Input: part model. Units: mm. Frame: model coordinates. A direction names the side the tool comes from. Coordinates: 2 decimals unless noted, no trailing zeros. Order: outer loops, then holes, each group sorted by start corner. A loop starts at its lowest first (then second) coordinate and runs counter-clockwise, first axis right, second up. Notation, with made-up numbers: M 14,50 L 62,50 A23 cw 62,84 Z; hole C 29.5,58 d6. An arc over 180 degrees is marked long. Answer in a Markdown table with one row per item.
from build123d import *

# Parameters (mm, degrees)
MAIN_BODY_DEPTH              = 34
SKETCH3_R                    = 3.571875
F_9_32_RIGHT_RAIL_DEPTH      = 1
F_9_32_RIGHT_RAIL_DEPTH_BACK = 39.1
SKETCH4_R                    = 3.571875
F_9_32_LEFT_RAIL_DEPTH       = 34
INNER_HOLLOW_DEPTH           = 21.3
SKETCH6_R                    = 3.571875
F_9_32_TOP_HOLE_DEPTH        = 1
F_9_32_TOP_HOLE_DEPTH_BACK   = 35


with BuildPart() as part:
    # Sketch1 → Main Body (new body)
    with BuildSketch(Plane(origin=(0, 0, 0), x_dir=(1, 0, 0), z_dir=(0, 1, 0))):
        Polygon((0, 0), (38.1, 0), (38.1, 9.525), (9.525, 38.1), (0, 38.1), align=None)
    extrude(amount=MAIN_BODY_DEPTH)

    # Sketch3 → 9/32 Right Rail (cut, two sides)
    with BuildSketch(Plane.XY) as f_9_32_right_rail_sk:
        with Locations((19.05, 17)):
            Circle(SKETCH3_R)
    extrude(amount=F_9_32_RIGHT_RAIL_DEPTH, mode=Mode.SUBTRACT)
    extrude(f_9_32_right_rail_sk.sketch, amount=-F_9_32_RIGHT_RAIL_DEPTH_BACK, mode=Mode.SUBTRACT)

    # Sketch4 → 9/32 Left Rail (cut)
    with BuildSketch(Plane.ZY):
        with Locations((-19.05, 17)):
            Circle(SKETCH4_R)
    extrude(amount=-F_9_32_LEFT_RAIL_DEPTH, mode=Mode.SUBTRACT)

    # Sketch5 → Inner Hollow (cut)
    with BuildSketch(Plane(origin=(0, 27.65, 0), x_dir=(1, 0, 0), z_dir=(0, 1, 0))):
        Polygon((3.175, 28.382403955), (11.208798023, 36.416201977), (36.416201977, 11.208798023), (28.382403955, 3.175), (3.175, 3.175), align=None)
    extrude(amount=-INNER_HOLLOW_DEPTH, mode=Mode.SUBTRACT)

    # Sketch6 → 9/32 Top Hole (cut, two sides)
    with BuildSketch(Plane(origin=(0, 34, 0), x_dir=(1, 0, 0), z_dir=(0, 1, 0))) as f_9_32_top_hole_sk:
        with Locations((11.90625, 11.90625)):
            Circle(SKETCH6_R)
    extrude(amount=F_9_32_TOP_HOLE_DEPTH, mode=Mode.SUBTRACT)
    extrude(f_9_32_top_hole_sk.sketch, amount=-F_9_32_TOP_HOLE_DEPTH_BACK, mode=Mode.SUBTRACT)


solid = part.part
1) Cut plane D-D, the plane z = -19.05. Output: boundary loops of the cut face in (x, y) (3 decimals), and give its area (3 significant figures).
Resolved:
| item | result |
|---|---|
| outline | M 0,0 L 28.575,0 L 28.575,6.35 L 3.175,6.35 L 3.175,13.428 L 0,13.428 Z; M 0,20.572 L 3.175,20.572 L 3.175,27.65 L 28.575,27.65 L 28.575,34 L 0,34 Z |
| area | 408 mm2 |
2) Cut plane B-B, the plane x = 17. Output: boundary loops of the cut face in (y, z) (3 decimals), and give its area (3 significant figures).
Resolved:
| item | result |
|---|---|
| outline | M 0,-30.625 L 6.35,-30.625 L 6.35,-3.175 L 14.075,-3.175 L 14.075,0 L 0,0 Z; M 19.925,-3.175 L 27.65,-3.175 L 27.65,-30.625 L 34,-30.625 L 34,0 L 19.925,0 Z |
| area | 438 mm2 |
3) Material intervals for probe 1 along Y at (x, z) = (13, -19); probe 2 along Y at (x, z) = (2, -19); probe 3 along X at (y, z) = (14.5, -12.5) (3 decimals), sorted ascending.
Resolved:
| item | result |
|---|---|
| probe 1 | y = 0 to 6.35, 27.65 to 34 |
| probe 2 | y = 0 to 13.43, 20.57 to 34 |
| probe 3 | x = 0 to 3.175 |
4) Reachability of faces 4 (the face through (7.136, 17.149, -32.343)), 5 (the face through (32.46, 17.15, -7.25)), 6 (the face through (16, 14.8, -3.175)) from +Z, -Z, +X, -X, +Y, -Y: full face, straight path, thin tool, end or side. Return the list, or none.
Resolved:
| item | result |
|---|---|
| face 4 | +X |
| face 5 | -Z |
| face 6 | none |
5) Mould query, pull axis Z, two halves, no side actions, for faces 1 (the face through (5, 17, -38.1)), 2 (the face through (3.175, 14.8, -15.6)), 3 (the face through (0, 13, -19)). Classes: +Z half, -Z half, draft (parallel to the pull), parting line (faces both ways), or undercut.
Resolved:
| item | result |
|---|---|
| face 1 | -Z half |
| face 2 | undercut |
| face 3 | draft |
6) Contact query for flat-ended pins moving along their axis: pin 1 (4 mm diameter, centred on x = 19, y = 19, fed in from -Z) (3 decimals); pin 2 (10.5 mm diameter, centred on x = 15.5, y = 17, fed in from -Z) (3 decimals); pin 3 (3 mm diameter, centred on y = 14, z = -27, fed in from +X). Output: stop coordinate, or through.
Resolved:
| item | result |
|---|---|
| pin 1 | stops at z = -3.175 |
| pin 2 | stops at z = -37.375 |
| pin 3 | stops at x = 3.29 |
7) Cut plane C-C, the plane z = -4. Output: boundary loops of the cut face in (x, y) (3 decimals), and give its area (3 significant figures).
Resolved:
| item | result |
|---|---|
| outline | M 0,0 L 38.1,0 L 38.1,34 L 0,34 Z; hole M 3.175,6.35 L 29.207,6.35 L 29.207,27.65 L 3.175,27.65 Z |
| area | 741 mm2 |
8) Cut plane A-A, the plane y = 17. Output: boundary loops of the cut face in (x, z) (3 decimals).
Resolved:
| item | result |
|---|---|
| outline | M 0,-38.1 L 9.525,-38.1 L 11.209,-36.416 L 3.175,-28.382 L 3.175,-22.622 L 0,-22.622 Z; M 0,-15.478 L 3.175,-15.478 L 3.175,-3.175 L 15.478,-3.175 L 15.478,0 L 0,0 Z; M 22.622,-3.175 L 28.382,-3.175 L 36.416,-11.209 L 38.1,-9.525 L 38.1,0 L 22.622,0 Z |
